Geometry: final body of the model. Coordinates: model frame, mm. A direction names the side the tool comes from. Give positions to 0.01 mm unless a question says otherwise; leave off trailing zeros. Write each loop counter-clockwise with the first axis right and the second up, starting at its lowest first coordinate (ties: lowest second). Pieces come first, ordered by that corner, then holes.
from build123d import *

# Parameters (mm, degrees)
SKETCH2_W                = 57
SKETCH2_H                = 57
SKETCH2_R                = 25.1
BOSS_EXTRUDE1_DEPTH      = 4.5
SKETCH2_3_R              = 25.1
SKETCH2_3_R_2            = 23.5
BOSS_EXTRUDE2_DEPTH      = 2
FILLET1_R                = 5
SKETCH4_R                = 2.5
SKETCH4_R_2              = 1.7
CUT_EXTRUDE1_DEPTH       = 41.555517504
BOSS_EXTRUDE3_DEPTH      = 1
FILLET2_R                = 0.2
CUT_EXTRUDE2_DEPTH       = 1.1
CIRPATTERN7_COUNT        = 4
FILLET2_OF_CIRPATTERN7_R = 0.2
FILLET3_R                = 5


with BuildPart() as part:
    # Sketch2 → Boss-Extrude1 (new body)
    with BuildSketch(Plane(origin=(0, 0, 0), x_dir=(1, 0, 0), z_dir=(0, 1, 0))):
        Rectangle(SKETCH2_W, SKETCH2_H)
        with Locations(Location((0, 0, 0), (0, 0, 270))):
            Circle(SKETCH2_R, mode=Mode.SUBTRACT)
    extrude(amount=BOSS_EXTRUDE1_DEPTH)

    # Sketch2_3 → Boss-Extrude2 (add)
    with BuildSketch(Plane(origin=(0, 0, 0), x_dir=(1, 0, 0), z_dir=(0, 1, 0))):
        with Locations(Location((0, 0, 0), (0, 0, 270))):
            Circle(SKETCH2_3_R)
        with Locations(Location((0, 0, 0), (0, 0, 270))):
            Circle(SKETCH2_3_R_2, mode=Mode.SUBTRACT)
    extrude(amount=BOSS_EXTRUDE2_DEPTH)

    # Fillet1
    fillet1_edges = [part.edges().sort_by_distance(p)[0] for p in [
        (-28.5, 2.25, -28.5),
    ]]
    fillet(fillet1_edges, radius=FILLET1_R)

    # Sketch4 → Cut-Extrude1 (cut, through all)
    with BuildSketch(Plane(origin=(0, 4.5, 0), x_dir=(1, 0, 0), z_dir=(0, 1, 0))):
        with Locations(Location((-23.5, 23.5, 0), (0, 0, 270))):
            Circle(SKETCH4_R)
        with Locations(Location((-15.5, 25, 0), (0, 0, 270))):
            Circle(SKETCH4_R_2)
    cut_extrude1 = extrude(amount=-CUT_EXTRUDE1_DEPTH, mode=Mode.SUBTRACT)

    # Sketch5 → Boss-Extrude3 (add)
    with BuildSketch(Plane(origin=(0, 4.5, 0), x_dir=(1, 0, 0), z_dir=(0, 1, 0))):
        Polygon((11, 27.5), (-11, 27.5), (-12, 28.5), (12, 28.5), align=None)
    boss_extrude3 = extrude(amount=BOSS_EXTRUDE3_DEPTH)

    # Fillet2
    fillet2_edges = [part.edges().sort_by_distance(p)[0] for p in [
        (0, 5.5, -27.5),
    ]]
    fillet(fillet2_edges, radius=FILLET2_R)

    # Sketch6 → Cut-Extrude2 (cut)
    with BuildSketch(Plane.XZ):
        Polygon((11, -27.5), (-11, -27.5), (-12, -28.5), (12, -28.5), align=None)
    cut_extrude2 = extrude(amount=-CUT_EXTRUDE2_DEPTH, mode=Mode.SUBTRACT)

    # CirPattern7: Cut-Extrude1, Boss-Extrude3, Cut-Extrude2 ×4 about axis
    cirpattern7_axis = Axis((0, 0, 0), (0, 1, 0))
    add([cut_extrude1.rotate(cirpattern7_axis, i * 360 / CIRPATTERN7_COUNT) for i in range(1, CIRPATTERN7_COUNT)], mode=Mode.SUBTRACT)
    add([boss_extrude3.rotate(cirpattern7_axis, i * 360 / CIRPATTERN7_COUNT) for i in range(1, CIRPATTERN7_COUNT)])
    add([cut_extrude2.rotate(cirpattern7_axis, i * 360 / CIRPATTERN7_COUNT) for i in range(1, CIRPATTERN7_COUNT)], mode=Mode.SUBTRACT)

    # Fillet2 of CirPattern7
    fillet2_of_cirpattern7_edges = [part.edges().sort_by_distance(p)[0] for p in [
        (-27.5, 5.5, 0),
        (0, 5.5, 27.5),
        (27.5, 5.5, 0),
    ]]
    fillet(fillet2_of_cirpattern7_edges, radius=FILLET2_OF_CIRPATTERN7_R)

    # Fillet3
    fillet3_edges = [part.edges().sort_by_distance(p)[0] for p in [
        (28.5, 2.25, -28.5),
        (28.5, 2.25, 28.5),
        (-28.5, 2.25, 28.5),
    ]]
    fillet(fillet3_edges, radius=FILLET3_R)


solid = part.part
Q1. Access query for faces 4 (the flat face through (-26, 4.5, 0)), 5 (the flat face through (0, 3, -28.5)). Directions: +Z, -Z, +X, -X, +Y, -Y. A direction counts if a zero-diameter tool reaches every point of the face in a straight line with its end or side. Return the directions, or none.
Filled sheet:
face 4: +Y
face 5: -Z, +X, -X, +Y, -Y
Q2. Section C-C on x = 15.5. Output: boundary loops of the cut face in (y, z), plus the area to 3 significant figures.
Filled sheet:
outline: (0, -28.5) - (4.5, -28.5) - (4.5, -19.74) - (2, -19.74) - (2, -17.66) - (0, -17.66) - close; (0, 17.66) - (2, 17.66) - (2, 19.74) - (4.5, 19.74) - (4.5, 23.3) - (0, 23.3) - close; (0, 26.7) - (4.5, 26.7) - (4.5, 28.5) - (0, 28.5) - close
area: 71.8 mm2
Q3. Section D-D on x = 9. Output: boundary loops of the cut face in (y, z), plus the area to 3 significant figures.
Filled sheet:
outline: (0, -27.5) - (1.1, -27.5) - (1.1, -28.5) - (5.5, -28.5) - (5.5, -27.7) arc R0.2 ccw to (5.3, -27.5) - (4.5, -27.5) - (4.5, -23.43) - (2, -23.43) - (2, -21.71) - (0, -21.71) - close; (0, 21.71) - (2, 21.71) - (2, 23.43) - (4.5, 23.43) - (4.5, 27.5) - (5.3, 27.5) arc R0.2 ccw to (5.5, 27.7) - (5.5, 28.5) - (1.1, 28.5) - (1.1, 27.5) - (0, 27.5) - close
area: 52.3 mm2
Q4. Section B-B on y = 3.55. Count the separate pieces of the cut face and the enclosed holes in it, plus the area to 3 significant figures.
Filled sheet:
separate pieces: 1
enclosed holes: 9
area: 1,130 mm2
Q5. Ray query, line 1 along Z through (x, y) = (7, 4.95); line 2 along Z through (x, y) = (-21.5, 0.75); line 3 along Z through (x, y) = (0.5, 1.75). Return the intervals inside material, ascending.
Filled sheet:
line 1: z = -28.5 to -27.5, 27.5 to 28.5
line 2: z = -28.5 to -25, -22 to -9.49, 9.49 to 22, 25 to 28.5
line 3: z = -28.5 to -23.49, 23.49 to 28.5
Q6. Pull-direction query (X, two-part tool) for faces 1 (the cylindrical face through (23.83, 2.28, -21.02)), 2 (the flat face through (-28.5, 3, 0)), 3 (the cylindrical face through (27.07, 2.28, -27)); classes: released by +X, released by -X, zero draft, split by the parting line, or undercut.
Filled sheet:
face 1: undercut
face 2: released by -X
face 3: released by +X
Q7. Pin query (flat end, axial travel): P1, Ø0.9, axis at y = 0.5, z = 4, coming from the -X side; P2, Ø6, axis at x = -23.5, z = -23.5, coming from the +Y side. Return the tip coordinate at first contact, or that it passes through.
Filled sheet:
P1: stops at x = -27.5
P2: stops at y = 4.5
Q8. Section A-A on z = 0. Output: boundary loops of the cut face in (x, y).
Filled sheet:
outline: (-28.5, 1.1) - (-27.5, 1.1) - (-27.5, 0) - (-23.5, 0) - (-23.5, 2) - (-25.1, 2) - (-25.1, 4.5) - (-27.5, 4.5) - (-27.5, 5.3) arc R0.2 ccw to (-27.7, 5.5) - (-28.5, 5.5) - close; (23.5, 0) - (27.5, 0) - (27.5, 1.1) - (28.5, 1.1) - (28.5, 5.5) - (27.7, 5.5) arc R0.2 ccw to (27.5, 5.3) - (27.5, 4.5) - (25.1, 4.5) - (25.1, 2) - (23.5, 2) - close
